Verification items for the finished model (mm, model axes). A direction names the side the tool comes from. Give positions to 0.01 mm unless a question says otherwise; leave off trailing zeros. Loops run counter-clockwise (first coordinate to the right, second up) from the corner with the lowest first, then second, coordinate; pieces in that order, holes last. Notation, with made-up numbers: (43, 60.5) -> (81, 60.5) arc R18 ccw to (81, 91.5) -> close; hole circle Ø7 at (51.5, 9.5). An arc over 180 degrees is marked (long way). Answer in a Markdown table with one row per item. Add a question column.
Q1. Set-up check for faces 1 (the face through (-25.38, -6.68, -7.01)), 2 (the face through (-26, 5.4, -6)), 3 (the face through (-23, 7, -10)), 4 (the face through (-19, -2.5, 4)): record each of +Z, -Z, +X, -X, +Y, -Y from which the full face is reachable in a straight line by a thin tool's end or side.
Q2. Section check C-C on y = -0.25. Enter the section's corners in (x, z), and give its area (3 significant figures).
Q3. Gauge pin test, flat ends, axial feed: P1, Ø4, axis at x = 27, z = -8.5, coming from the +Y side; P2, Ø3, axis at x = -1, y = 1, coming from the -Z side. Record the tip position at first contact, or that the pin passes through.
Q4. Section check A-A on z = -8.5. Give the number of separate pieces and of enclosed holes in the cut face, and give its area (3 significant figures).
Q5. Release check for a two-part mould opening along Y. For faces 5 (the face through (-23, 0, 4)), 6 (the face through (0, -8, 2)), 7 (the face through (-25.38, 6.72, -7.01)) record: pulls with the +Y half, pulls with the -Y half, needs draft (parallel to the pull), parting line crosses it, or undercut.
Q6. Section check D-D on x = -27. Enter the section's corners in (y, z).
Q7. Section check B-B on x = 20. Enter the section's corners in (y, z), and give its area (3 significant figures).
Q8. Material ranges on probe 1 along X at (y, z) = (-1.75, 2.75); probe 2 along Y at (x, z) = (22, 1.5); probe 3 along Y at (x, z) = (29, -3), recorded low to high.
```python
from build123d import *

# Parameters (mm, degrees)
SKETCH_W        = 64
SKETCH_H        = 16
PAD_DEPTH       = 8
SKETCH001_W     = 15
SKETCH001_H     = 2.6
PAD001_DEPTH    = 15
SKETCH002_R     = 2.2
POCKET_DEPTH    = 16
CHAMFER_SIZE    = 11
CHAMFER001_SIZE = 11
CHAMFER002_SIZE = 11
CHAMFER003_SIZE = 11
FILLET_R        = 3.9
FILLET001_R     = 3.9
FILLET002_R     = 3.9
FILLET003_R     = 3.9
SKETCH004_W     = 8
SKETCH004_H     = 5
POCKET001_DEPTH = 8


with BuildPart() as part:
    # Sketch → Pad (new body)
    with BuildSketch(Plane.XY):
        Rectangle(SKETCH_W, SKETCH_H)
    extrude(amount=PAD_DEPTH)

    # Sketch001 (on Face5 of Pad) → Pad001 (join)
    with BuildSketch(Plane(origin=(0, 0, 0), x_dir=(1, 0, 0), z_dir=(0, 0, -1))):
        with Locations((-24.5, 6.7)):
            Rectangle(SKETCH001_W, SKETCH001_H)
        with Locations((-24.5, -6.7)):
            Rectangle(SKETCH001_W, SKETCH001_H)
        with Locations((24.5, 6.7)):
            Rectangle(SKETCH001_W, SKETCH001_H)
        with Locations((24.5, -6.7)):
            Rectangle(SKETCH001_W, SKETCH001_H)
    extrude(amount=PAD001_DEPTH)

    # Sketch002 (on Face4 of Pad001) → Pocket (cut)
    with BuildSketch(Plane(origin=(0, 8, 0), x_dir=(-1, 0, 0), z_dir=(0, 1, 0))):
        with Locations((-27, -8.5)):
            Circle(SKETCH002_R)
        with Locations((27, -8.5)):
            Circle(SKETCH002_R)
    extrude(amount=-POCKET_DEPTH, mode=Mode.SUBTRACT)

    # Chamfer
    chamfer_edges = [part.edges().sort_by_distance(p)[0] for p in [
        (17, 6.7, -15),
    ]]
    chamfer(chamfer_edges, length=CHAMFER_SIZE)

    # Chamfer001
    chamfer001_edges = [part.edges().sort_by_distance(p)[0] for p in [
        (17, -6.7, -15),
    ]]
    chamfer(chamfer001_edges, length=CHAMFER001_SIZE)

    # Chamfer002
    chamfer002_edges = [part.edges().sort_by_distance(p)[0] for p in [
        (-17, 6.7, -15),
    ]]
    chamfer(chamfer002_edges, length=CHAMFER002_SIZE)

    # Chamfer003
    chamfer003_edges = [part.edges().sort_by_distance(p)[0] for p in [
        (-17, -6.7, -15),
    ]]
    chamfer(chamfer003_edges, length=CHAMFER003_SIZE)

    # Fillet
    fillet_edges = [part.edges().sort_by_distance(p)[0] for p in [
        (-32, 6.7, -15),
    ]]
    fillet(fillet_edges, radius=FILLET_R)

    # Fillet001
    fillet001_edges = [part.edges().sort_by_distance(p)[0] for p in [
        (-32, -6.7, -15),
    ]]
    fillet(fillet001_edges, radius=FILLET001_R)

    # Fillet002
    fillet002_edges = [part.edges().sort_by_distance(p)[0] for p in [
        (32, -6.7, -15),
    ]]
    fillet(fillet002_edges, radius=FILLET002_R)

    # Fillet003
    fillet003_edges = [part.edges().sort_by_distance(p)[0] for p in [
        (32, 6.7, -15),
    ]]
    fillet(fillet003_edges, radius=FILLET003_R)

    # Sketch004 (on Face21 of Fillet003) → Pocket001 (cut)
    with BuildSketch(Plane.XY.offset(8)):
        with Locations((-19, 0)):
            Rectangle(SKETCH004_W, SKETCH004_H)
        with Locations((19, 0)):
            Rectangle(SKETCH004_W, SKETCH004_H)
    extrude(amount=-POCKET001_DEPTH, mode=Mode.SUBTRACT)


solid = part.part
```
Taken from the geometry:
| question | item | result |
|---|---|---|
| 1 | face 1 | +Y, -Y |
| 1 | face 2 | -Z, +X, -X |
| 1 | face 3 | -Z, +Y, -Y |
| 1 | face 4 | +Z, -Z |
| 2 | outline | (-32, 0) -> (-23, 0) -> (-23, 8) -> (-32, 8) -> close; (-15, 0) -> (15, 0) -> (15, 8) -> (-15, 8) -> close; (23, 0) -> (32, 0) -> (32, 8) -> (23, 8) -> close |
| 2 | area | 384 mm² |
| 3 | P1 | passes through |
| 3 | P2 | stops at z = 0 |
| 4 | separate pieces | 8 |
| 4 | enclosed holes | 0 |
| 4 | area | 63.4 mm² |
| 5 | face 5 | undercut |
| 5 | face 6 | pulls with the -Y half |
| 5 | face 7 | needs draft |
| 6 | outline | (-8, -14) -> (-5.4, -14) -> (-5.4, -10.7) -> (-8, -10.7) -> close; (-8, -6.3) -> (-5.4, -6.3) -> (-5.4, 0) -> (5.4, 0) -> (5.4, -6.3) -> (8, -6.3) -> (8, 8) -> (-8, 8) -> close; (5.4, -14) -> (8, -14) -> (8, -10.7) -> (5.4, -10.7) -> close |
| 7 | outline | (-8, -7) -> (-5.4, -7) -> (-5.4, 0) -> (-2.5, 0) -> (-2.5, 8) -> (-8, 8) -> close; (2.5, 0) -> (5.4, 0) -> (5.4, -7) -> (8, -7) -> (8, 8) -> (2.5, 8) -> close |
| 7 | area | 124 mm² |
| 8 | probe 1 | x = -32 to -23, -15 to 15, 23 to 32 |
| 8 | probe 2 | y = -8 to -2.5, 2.5 to 8 |
| 8 | probe 3 | y = -8 to -5.4, 5.4 to 8 |
